```python
from build123d import *

# Parameters (mm, degrees)
SKETCH_1_W      = 40
SKETCH_1_H      = 56
EXTRUDE_1_DEPTH = 3
HOLE_WIZARD_1_D = 2.4
EXTRUDE_2_DEPTH = 4


with BuildPart() as part:
    # 草图1 → 凸台-拉伸1 (new body)
    with BuildSketch(Plane(origin=(0, 0, 0), x_dir=(1, 0, 0), z_dir=(0, 1, 0))):
        Rectangle(SKETCH_1_W, SKETCH_1_H)
    extrude(amount=EXTRUDE_1_DEPTH)

    # 孔1 (through all)
    with Locations(Plane(origin=(0, 3, 0), x_dir=(1, 0, 0), z_dir=(0, 1, 0))):
        with Locations((-18, 10.2), (18, 10.2), (18, -25.8), (-18, -25.8)):
            Hole(HOLE_WIZARD_1_D / 2)

    # 草图5 → 凸台-拉伸2 (add)
    with BuildSketch(Plane(origin=(0, 3, 0), x_dir=(1, 0, 0), z_dir=(0, 1, 0))):
        Polygon((-7, 28), (-7, 18), (7, 18), (7, 28), (0, 28), align=None)
    extrude(amount=EXTRUDE_2_DEPTH)


solid = part.part
```
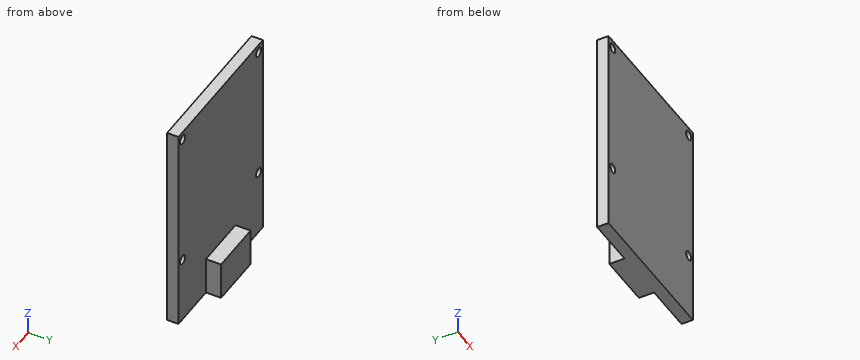
Could you check a few things on this model? Use its own coordinates, in mm. Round coordinates to 2 decimals unless told otherwise and drop trailing zeros. Order: outer loops, then holes, each group sorted by start corner. A loop starts at its lowest first (then second) coordinate and runs counter-clockwise, first axis right, second up. Notation, with made-up numbers: (-31.5, -30.5) -> (5.5, -30.5) arc R15 cw to (5.5, -4.5) -> close; hole circle Ø8 at (-26, 82). An arc over 180 degrees is marked (long way). One line per question, with ' | ' between items.
Q1. If we section it at A-A on z = -10.2: Write out the boundary of the cut face in (x, y).
Computed values:
outline: (-20, 0) -> (-19.2, 0) -> (-19.2, 3) -> (-20, 3) -> close; (-16.8, 0) -> (16.8, 0) -> (16.8, 3) -> (-16.8, 3) -> close; (19.2, 0) -> (20, 0) -> (20, 3) -> (19.2, 3) -> close
Q2. If we section it at D-D on x = -3: Write out the boundary of the cut face in (y, z), plus the area to 3 significant figures.
Computed values:
outline: (0, -28) -> (7, -28) -> (7, -18) -> (3, -18) -> (3, 28) -> (0, 28) -> close | area: 208 mm²
Q3. I'm going to push flat-ended pins straight in: pin 1 (1.2 mm diameter, centred on y = 5.5, z = -22.5, fed in from -X); pin 2 (12 mm diameter, centred on x = -8, z = -7, fed in from +Y); pin 3 (1.2 mm diameter, centred on y = 5.5, z = -21.5, fed in from +X). Where does each tip first touch, or does it pass through?
Computed values:
pin 1: x = -7 | pin 2: y = 3 | pin 3: x = 7
Q4. If we section it at B-B on x = -18: Write out the boundary of the cut face in (y, z), plus the area to 3 significant figures.
Computed values:
outline: (0, -28) -> (3, -28) -> (3, -11.4) -> (0, -11.4) -> close; (0, -9) -> (3, -9) -> (3, 24.6) -> (0, 24.6) -> close; (0, 27) -> (3, 27) -> (3, 28) -> (0, 28) -> close | area: 154 mm²
Q5. If we section it at C-C on y = 4: Write out the boundary of the cut face in (x, z), plus the area to 3 significant figures.
Computed values:
outline: (-7, -28) -> (7, -28) -> (7, -18) -> (-7, -18) -> close | area: 140 mm²
Q6. If I drill on line 1 (X direction, y = 0.95, z = -10.2); line 2 (Z direction, x = -18, y = 1.95); line 3 (Z direction, x = -17, y = 1.25), over which ranges is the centre line in solid material (lowest first)? Write a range as from..to.
Computed values:
line 1: -20..-19.2, -16.8..16.8, 19.2..20 | line 2: -28..-11.4, -9..24.6, 27..28 | line 3: -28..-10.86, -9.54..25.14, 26.46..28
